Autodesk Inventor part; units mm, degrees
ref_plane "YZ Plane" through (0, 0, 0) normal (1, 0, 0) x (0, 1, 0)
ref_plane "XZ Plane" through (0, 0, 0) normal (0, 1, 0) x (-1, 0, 0)
ref_plane "XY Plane" through (0, 0, 0) normal (0, 0, 1) x (1, 0, 0)
sketch "Sketch1" plane through (0, 0, 0) normal (0, 1, 0) x (-1, 0, 0)
  circle A0 centre (0, 0) radius 5.08
  dimension "d0" = 10.16
extrude "Extrusion1" add sketch "Sketch1" along normal blind 101.6
sketch "Sketch2" plane through (0, 101.6, 0) normal (0, 1, 0) x (1, 0, 0)
  circle A0 centre (0, 0) radius 5.08
  line L0 (0, 0) -> (-2.54, 0)
  line L1 (38.1, 0) -> (40.64, 0)
  arc A1 (38.1, 0) -> (0, 0) centre (19.05, 0) ccw
  arc A2 (40.64, 0) -> (-2.54, 0) centre (19.05, 0) ccw
  line L2 (38.1, 0) -> (40.64, 0) construction
  line L3 (5.08, 0) -> (-2.54, 0) construction
  line L4 (-2.54, 0) -> (5.08, 0)
  line L5 (38.1, 0) -> (40.64, 0)
  dimension "d64" = 2.54
  dimension "d65" = 2.54
  dimension "d66" = 38.1
  dimension "d67" = 19.05
  dimension "d68" = 180
  dimension "d69" = 21.59
extrude "Extrusion5" add sketch "Sketch2" against normal blind 6.35 contours A1 L0 A2 A0 | A0 A2 L1 A1
sketch "Sketch4" plane through (0, 0, 0) normal (0, -1, 0) x (1, 0, 0)
  circle A0 centre (0, 0) radius 9.525
  dimension "d72" = 19.05
extrude "Extrusion6" add sketch "Sketch4" along normal blind 3.175
sketch "Sketch5" plane through (0, -3.175, 0) normal (0, -1, 0) x (1, 0, 0)
  point P0 (0, 0)
  point P1 (0, 8.001)
  point P2 (0, -8.001)
  point P3 (8.001, 0)
  point P4 (-8.001, 0)
  dimension "d79" = 8.001
  dimension "d80" = 8.001
  dimension "d81" = 8.001
  dimension "d82" = 8.001
hole "Hole1" at (0, -3.175, 8.001) at (0, -3.175, -8.001) at (8.001, -3.175, 0) at (-8.001, -3.175, 0) direction (0, 1, 0) diameter 2.4892 depth 25.4 tip angle 118
ref_plane "Work Plane6" through (0, 66.675, 0) normal (0, 1, 0) x (1, 0, 0)
sketch "Sketch6" plane through (0, 66.675, 0) normal (0, 1, 0) x (1, 0, 0)
  line L0 (0, 0) -> (1.27, 0)
  line L1 (1.27, 0) -> (-1.27, 0)
  arc A0 (38.1, 0) -> (0.6773, 5.0346) centre (19.05, 0) ccw
  arc A1 (1.27, 0) -> (36.83, 0) centre (19.05, 0) ccw
  arc A2 (-1.27, 0) -> (39.37, 0) centre (19.05, 0) ccw
  line L2 (39.37, 0) -> (36.83, 0)
  line L3 (1.27, 0) -> (-1.27, 0)
  dimension "d91" = 1.27
  dimension "d92" = 2.54
properties part number "pincherleft"
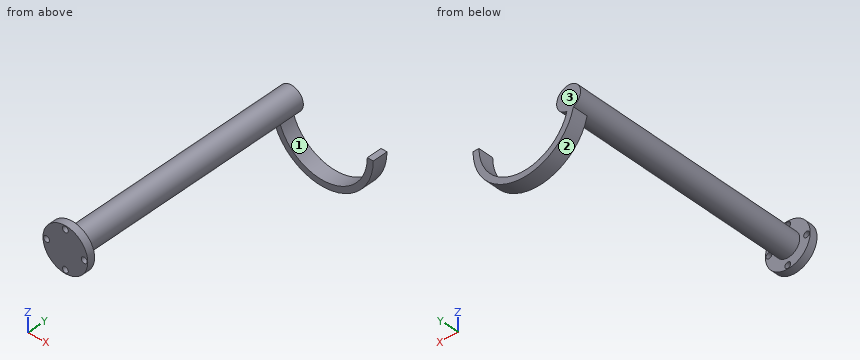
Geometry check sheet. Reference: the model listing, model coordinates, mm. Face numbers are marked on the shaded views. Round coordinates to 2 decimals unless told otherwise and drop trailing zeros. Loops run counter-clockwise (first coordinate to the right, second up) from the corner with the lowest first, then second, coordinate; pieces in that order, holes last. Notation, with made-up numbers: (-23, 77) - (20, 77) arc R23 ccw to (20, 116) - close; hole circle Ø7 at (0.5, 88). An arc over 180 degrees is marked (long way). Write each question's results on one line, items separated by ' | '. Start each with the question number.
Q1. Thickness scan on line 1 (Z direction, x = 0, y = -1.7) (3 decimals); line 2 (Y direction, x = -7, z = 6) (3 decimals); line 3 (Y direction, x = 4.5, z = -15.5). Record the ranges inside material, lowest first. Write a range as [from, to].
Q2. Gauge pin test, flat ends, axial feed: P1, Ø1.5, axis at y = 19.5, z = 0.5, coming from the +X side; P2, Ø3, axis at x = -8.001, z = 0, coming from the +Y side; P3, Ø1.5, axis at x = 0, z = -8.001, coming from the -Y side. Record the tip position at first contact, or that the pin passes through.
Q3. Release check for a two-part mould opening along X. For the marked faces 1, 2 and 3 record: +X half, -X half, draft (parallel to the pull), parting line (faces both ways), or undercut.
Q4. Cross-section at C-C on z = 4. Enter the section's corners in (x, y) (3 decimals).
Q5. Cross-section at A-A on z = -17.5. Enter the section's corners in (x, y).
Q6. Cross-section at B-B on y = 34. Enter the section's corners in (x, z).
Answers below:
1) line 1: z = [-9.525, -9.246], [-6.756, 6.756], [9.246, 9.525] | line 2: y = [-3.175, 0] | line 3: y = [95.25, 101.6]
2) P1: stops at x = 5.08 | P2: stops at y = 0 | P3: stops at y = 95.25
3) face 1: undercut | face 2: parting line | face 3: draft
4) outline: (-8.644, -3.175) - (8.644, -3.175) - (8.644, 0) - (3.132, 0) - (3.132, 101.6) - (-3.132, 101.6) - (-3.132, 0) - (-8.644, 0) - close
5) outline: (6.41, 95.25) - (11.52, 95.25) - (11.52, 101.6) - (6.41, 101.6) - close; (26.58, 95.25) - (31.69, 95.25) - (31.69, 101.6) - (26.58, 101.6) - close
6) outline: circle Ø10.16 at (0, 0)
